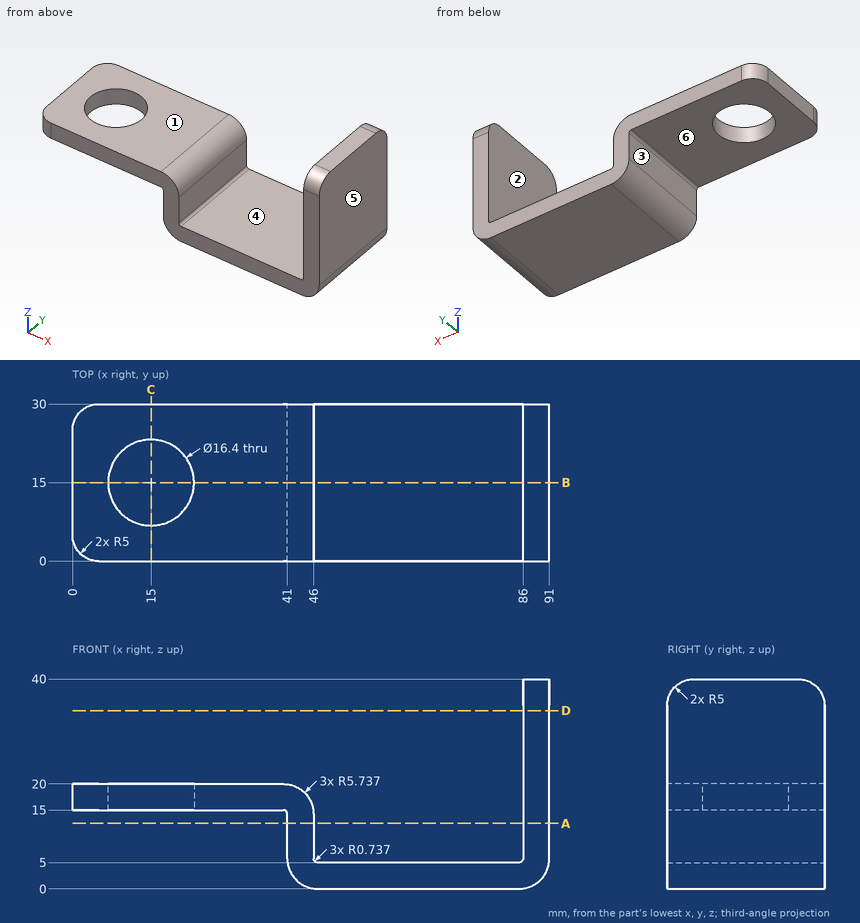
Check sheet for the drawn part. Datum: minimum x, y, z corner. Units: mm. A direction names the side the tool comes from. Give positions to 0.01 mm unless a question says otherwise; leave off trailing zeros. Write each loop counter-clockwise with the first axis right and the second up, starting at its lowest first coordinate (ties: lowest second). Pieces come first, ordered by that corner, then holes. Notation, with made-up numbers: M -7.75,-35.75 L 17.25,-35.75 A19 cw 17.25,-22.75 Z; hole C 30,14.25 d4. An arc over 180 degrees is marked long. One line per question, with ' | ' between items.
1) Set-up check for the marked faces 4, 5 and 6: record each of +Z, -Z, +X, -X, +Y, -Y from which the full face is reachable in a straight line by a thin tool's end or side.
Result:
face 4: +Z, +Y, -Y | face 5: +Z, -Z, +X, +Y, -Y | face 6: -Z, -X, +Y, -Y
2) Section check D-D on z = 34. Enter the section's corners in (x, y), plus the area to 3 significant figures.
Result:
outline: M 86,0 L 91,0 L 91,30 L 86,30 Z | area: 150 mm2
3) Section check C-C on x = 15. Enter the section's corners in (y, z).
Result:
outline: M 0,15 L 6.8,15 L 6.8,20 L 0,20 Z; M 23.2,15 L 30,15 L 30,20 L 23.2,20 Z
4) Section check B-B on y = 15. Enter the section's corners in (x, z).
Result:
outline: M 0,15 L 6.8,15 L 6.8,20 L 0,20 Z; M 23.2,15 L 40.26,15 A0.74 cw 41,14.26 L 41,5.74 A5.74 ccw 46.74,0 L 85.26,0 A5.74 ccw 91,5.74 L 91,40 L 86,40 L 86,5.74 A0.74 cw 85.26,5 L 46.74,5 A0.74 cw 46,5.74 L 46,14.26 A5.74 ccw 40.26,20 L 23.2,20 Z
5) Thickness scan on line 1 along X through (y, z) = (7.75, 7); line 2 along Y through (x, z) = (15, 18); line 3 along Z through (x, y) = (39, 23.5). Record the ranges inside material, lowest first. Write a range as [from, to].
Result:
line 1: x = [41, 46], [86, 91] | line 2: y = [0, 6.8], [23.2, 30] | line 3: z = [15, 20]
6) Gauge pin test, flat ends, axial feed: pin 1 Ø2 at (x, y) = (36.5, 24.5) entering from -Z; pin 2 Ø3 at (x, y) = (57, 21.5) entering from -Z; pin 3 Ø15 at (x, y) = (14.5, 21.5) entering from +Z; pin 4 Ø3 at (x, y) = (64, 13.5) entering from +Z. Record the tip position at first contact, or that the pin passes through.
Result:
pin 1: stops at z = 15 | pin 2: stops at z = 0 | pin 3: stops at z = 20 | pin 4: stops at z = 5
7) Mould release check, pull along X, two halves, no side actions. Record for the marked faces 1, 2 and 3: released by +X, released by -X, zero draft, split by the parting line, or undercut.
Result:
face 1: zero draft | face 2: undercut | face 3: released by -X
8) Section check A-A on z = 12.5. Enter the section's corners in (x, y), plus the area to 3 significant figures.
Result:
outline: M 41,0 L 46,0 L 46,30 L 41,30 Z; M 86,0 L 91,0 L 91,30 L 86,30 Z | area: 300 mm2
